Drawing for the job (mm, zero at the part's lowest x, y, z). A direction names the side the tool comes from. Coordinates: 2 decimals unless noted, no trailing zeros. Write each loop counter-clockwise with the first axis right and the second up, starting at its lowest first coordinate (ties: lowest second). Pieces come first, ordered by that corner, then holes. Notation, with made-up numbers: (16.5, 70) -> (53.5, 70) arc R34 ccw to (53.5, 105) -> close; hole circle Ø7 at (-19, 36). An arc over 180 degrees is marked (long way). Answer as CSV lines item,"result".
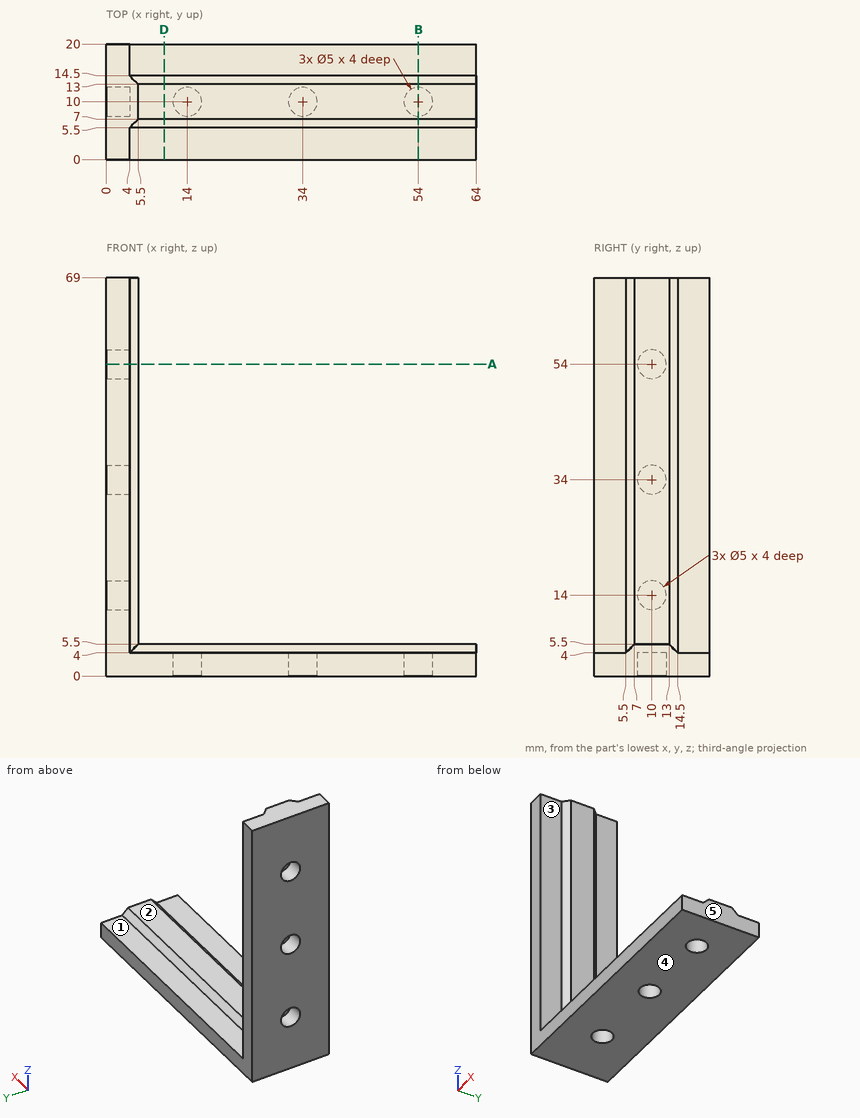
Item 1: Saw through at D-D on x = 10. Give the cut face in (y, z), and give its area (4 significant figures).
Answer below:
outline,"(0, 0) -> (20, 0) -> (20, 4) -> (14.5, 4) -> (13, 5.5) -> (7, 5.5) -> (5.5, 4) -> (0, 4) -> close"
area,"91.25 mm2"
Item 2: 3-axis set-ups, long thin cutter, end or side, ignore diameter. For the marked faces 1, 2, 3, 4 and 5: which of +Z, -Z, +X, -X, +Y, -Y reach the whole face in a straight line?
Answer below:
face 1,"+Z, +X, +Y"
face 2,"+Z, +X, +Y, -Y"
face 3,"+Z, +X, -Y"
face 4,"-Z, +X, -X, +Y, -Y"
face 5,"+Z, -Z, +X, +Y, -Y"
Item 3: Saw through at B-B on x = 54. Give the cut face in (y, z).
Answer below:
outline,"(0, 0) -> (7.5, 0) -> (7.5, 4) -> (12.5, 4) -> (12.5, 0) -> (20, 0) -> (20, 4) -> (14.5, 4) -> (13, 5.5) -> (7, 5.5) -> (5.5, 4) -> (0, 4) -> close"
Item 4: Saw through at A-A on z = 54. Give the cut face in (x, y), and give its area (4 significant figures).
Answer below:
outline,"(0, 0) -> (4, 0) -> (4, 5.5) -> (5.5, 7) -> (5.5, 13) -> (4, 14.5) -> (4, 20) -> (0, 20) -> (0, 12.5) -> (4, 12.5) -> (4, 7.5) -> (0, 7.5) -> close"
area,"71.25 mm2"
Item 5: Flat gauge pins, fed straight in: pin 1 (4.5 mm diameter, centred on x = 14, y = 10, fed in from +Z); pin 2 (3 mm diameter, centred on y = 10, z = 34, fed in from -X); pin 3 (1.5 mm diameter, centred on y = 9, z = 14, fed in from +X). Where does each tip first touch, or does it go through?
Answer below:
pin 1,"stops at z = 5.5"
pin 2,"stops at x = 4"
pin 3,"stops at x = 5.5"
Item 6: Wall check: line 1 (Z direction, x = 1.9, y = 10); line 2 (Y direction, x = 14, z = 2.05); line 3 (X direction, y = 3, z = 32). Give the ranges that are in metal, low to high. Write a range as from..to.
Answer below:
line 1,"z = 0..11.5, 16.5..31.5, 36.5..51.5, 56.5..69"
line 2,"y = 0..7.5, 12.5..20"
line 3,"x = 0..4"
